from build123d import *

# Parameters (mm, degrees)
SKETCH039_R             = 55
PAD008_DEPTH            = 10
POLARPATTERN003_COUNT   = 10
SKETCH040_R             = 55
SKETCH040_R_2           = 52.5
POCKET019_DEPTH         = 3
SKETCH041_R             = 1.75
POCKET020_DEPTH         = 321.770146
POCKET020_DEPTH_BACK    = 311.770146
POLARPATTERN004_COUNT   = 4
BODY002_PLACEMENT_ANGLE = 90


with BuildPart() as part:
    # Sketch039 → Pad008 (new body)
    with BuildSketch(Plane.XZ):
        Circle(SKETCH039_R)
        with BuildLine():
            ThreePointArc((49.807718, 4.380782), (-50, 0), (49.807718, -4.380782))
            ThreePointArc((49.807718, 4.380782), (45.615, 0), (49.807718, -4.380782))
        make_face(mode=Mode.SUBTRACT)
    pad008 = extrude(amount=PAD008_DEPTH)

    # PolarPattern003: Pad008 ×10 about axis
    polarpattern003_axis = Axis((0, 0, 0), (0, -1, 0))
    for i in range(1, POLARPATTERN003_COUNT):
        add(pad008.rotate(polarpattern003_axis, i * 360 / POLARPATTERN003_COUNT))

    # Sketch040 (on DatumPlane) → Pocket019 (cut)
    with BuildSketch(Plane.XZ.offset(10)):
        Circle(SKETCH040_R)
        Circle(SKETCH040_R_2, mode=Mode.SUBTRACT)
    extrude(amount=-POCKET019_DEPTH, mode=Mode.SUBTRACT)

    # Sketch041 (on DatumPlane) → Pocket020 (cut, two sides)
    with BuildSketch(Plane.XZ.offset(10)) as pocket020_sk:
        with Locations((52.5, 0)):
            Circle(SKETCH041_R)
    pocket020 = extrude(amount=-POCKET020_DEPTH, mode=Mode.SUBTRACT) + extrude(pocket020_sk.sketch, amount=POCKET020_DEPTH_BACK, mode=Mode.SUBTRACT)

    # PolarPattern004: Pocket020 ×4 about axis
    polarpattern004_axis = Axis((0, -10, 0), (0, -1, 0))
    for i in range(1, POLARPATTERN004_COUNT):
        add(pocket020.rotate(polarpattern004_axis, i * 360 / POLARPATTERN004_COUNT), mode=Mode.SUBTRACT)


with BuildPart() as part_1:
    # Body002 placement: moved
    add(part.part.moved(Location((-1.52, 0, 16))).rotate(Axis((-1.52, 0, 16), (1, 0, 0)), BODY002_PLACEMENT_ANGLE))


solid = part_1.part
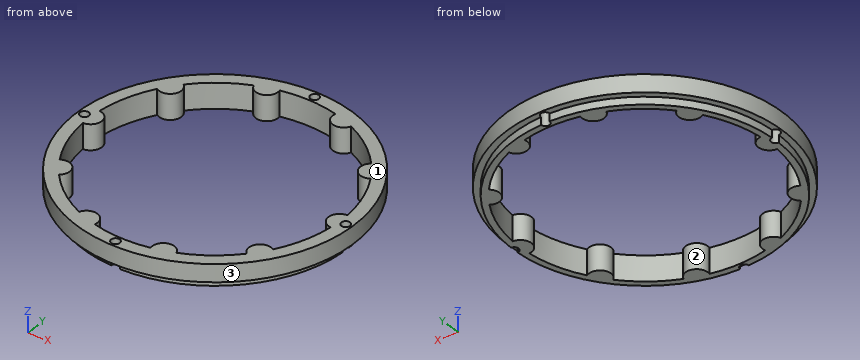
Verification items for the finished model (mm, model axes). Face numbers are marked on the shaded views. Give positions to 0.01 mm unless a question says otherwise; leave off trailing zeros. Loops run counter-clockwise (first coordinate to the right, second up) from the corner with the lowest first, then second, coordinate; pieces in that order, holes last.
1. Go/stop test with flat-tipped pins: P1, Ø4, axis at y = 29, z = 11.5, coming from the +X side; P2, Ø4, axis at y = -18, z = 14.5, coming from the +X side; P3, Ø3, axis at x = -15.5, z = 10.5, coming from the +Y side; P4, Ø1.5, axis at x = 42, y = -1, coming from the +Z side. Record where each tip stops, or that it passes through.
Derived:
P1: stops at x = 46.4
P2: stops at x = 51.1
P3: stops at y = 53.57
P4: passes through
2. Cross-section at C-C on x = -1.52. Record the cut outline in (y, z), and give its area (3 significant figures).
Derived:
outline: (-55, 9) - (-54.25, 9) - (-54.25, 16) - (-55, 16) - close; (-50.75, 6) - (-50, 6) - (-50, 16) - (-50.75, 16) - close; (50, 6) - (50.75, 6) - (50.75, 16) - (50, 16) - close; (54.25, 9) - (55, 9) - (55, 16) - (54.25, 16) - close
area: 25.5 mm2
3. Cross-section at B-B on z = 7.25. Record the cut outline in (x, y) (3 decimals), and give its area (3 significant figures).
Derived:
outline: (-53.991, -1.75) arc R52.5 ccw to (-3.27, -52.471) arc R1.75 cw to (0.23, -52.471) arc R52.5 ccw to (50.951, -1.75) arc R1.75 cw to (50.951, 1.75) arc R52.5 ccw to (0.23, 52.471) arc R1.75 cw to (-3.27, 52.471) arc R52.5 ccw to (-53.991, 1.75) arc R1.75 cw to start; hole (-51.328, -4.381) arc R50 ccw to (-44.39, -25.732) arc R4.385 cw to (-39.24, -32.82) arc R50 ccw to (-21.078, -46.016) arc R4.385 cw to (-12.745, -48.724) arc R50 ccw to (9.705, -48.724) arc R4.385 cw to (18.038, -46.016) arc R50 ccw to (36.2, -32.82) arc R4.385 cw to (41.35, -25.732) arc R50 ccw to (48.288, -4.381) arc R4.385 cw to (48.288, 4.381) arc R50 ccw to (41.35, 25.732) arc R4.385 cw to (36.2, 32.82) arc R50 ccw to (18.038, 46.016) arc R4.385 cw to (9.705, 48.724) arc R50 ccw to (-12.745, 48.724) arc R4.385 cw to (-21.078, 46.016) arc R50 ccw to (-39.24, 32.82) arc R4.385 cw to (-44.39, 25.732) arc R50 ccw to (-51.328, 4.381) arc R4.385 cw to start
area: 1,080 mm2
4. Cross-section at D-D on x = -16. Record the cut outline in (y, z).
Derived:
outline: (-53.06, 9) - (-50.46, 9) - (-50.46, 6) - (-43.28, 6) - (-43.28, 16) - (-53.06, 16) - close; (43.28, 6) - (50.46, 6) - (50.46, 9) - (53.06, 9) - (53.06, 16) - (43.28, 16) - close
5. Material ranges on probe 1 along X at (y, z) = (0, 14) (3 decimals); probe 2 along Y at (x, z) = (-26.5, 14.5); probe 3 along Y at (x, z) = (-17.5, 15.25), recorded low to high.
Derived:
probe 1: x = -56.52 to -55.77, -52.27 to -47.135, 44.095 to 49.23, 52.73 to 53.48
probe 2: y = -49 to -43.31, 43.31 to 49
probe 3: y = -52.63 to -43.2, 43.2 to 52.63
6. Cross-section at A-A on y = 0. Record the cut outline in (x, z) (3 decimals).
Derived:
outline: (-56.52, 9) - (-55.77, 9) - (-55.77, 16) - (-56.52, 16) - close; (-52.27, 6) - (-47.135, 6) - (-47.135, 16) - (-52.27, 16) - close; (44.095, 6) - (49.23, 6) - (49.23, 16) - (44.095, 16) - close; (52.73, 9) - (53.48, 9) - (53.48, 16) - (52.73, 16) - close
7. Release check for a two-part mould opening along Y. For the marked faces 1, 2 and 3 record: +Y half, -Y half, draft (parallel to the pull), parting line (faces both ways), or undercut.
Derived:
face 1: draft
face 2: undercut
face 3: parting line
